Answer from the drawing. Dimensions are ordinates in mm from the lowest x, y and z of the part. A direction names the side the tool comes from. Coordinates: 2 decimals unless noted, no trailing zeros. Write each loop counter-clockwise with the first axis right and the second up, starting at its lowest first coordinate (ties: lowest second). Pieces come first, ordered by that corner, then holes. Notation, with made-up numbers: (10.5, 13) -> (56.5, 13) arc R13 cw to (56.5, 27) -> close; hole circle Ø11 at (16.5, 62.25). An arc over 180 degrees is marked (long way). Return JSON: item names as keys, results as strings.
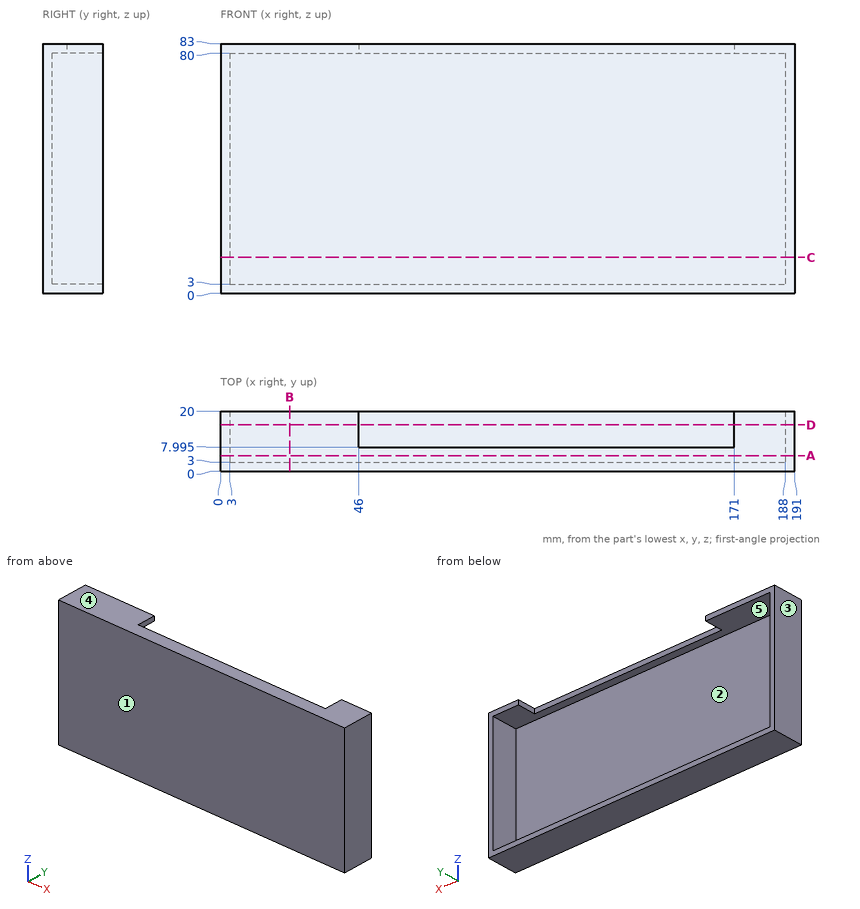
1. The part is cut by section D-D (y = 15.5). Determine the outline of the cut face in (x, z), then the cut area to 3 significant figures.
Taken from the geometry:
{"outline": "(0, 0) -> (191, 0) -> (191, 83) -> (171, 83) -> (171, 80) -> (188, 80) -> (188, 3) -> (3, 3) -> (3, 80) -> (46, 80) -> (46, 83) -> (0, 83) -> close", "area": "1,230 mm2"}
2. The part is cut by section C-C (z = 12). Determine the outline of the cut face in (x, y), then the cut area to 3 significant figures.
Taken from the geometry:
{"outline": "(0, 0) -> (191, 0) -> (191, 20) -> (188, 20) -> (188, 3) -> (3, 3) -> (3, 20) -> (0, 20) -> close", "area": "675 mm2"}
3. The part is cut by section B-B (x = 23). Determine the outline of the cut face in (y, z).
Taken from the geometry:
{"outline": "(0, 0) -> (20, 0) -> (20, 3) -> (3, 3) -> (3, 80) -> (20, 80) -> (20, 83) -> (0, 83) -> close"}
4. For a pull along X with two mould halves and no side action, classify the marked faces 1, 2 and 3 as +X half, -X half, draft (parallel to the pull), parting line (faces both ways), or undercut.
Taken from the geometry:
{"face 1": "draft", "face 2": "undercut", "face 3": "-X half"}
5. A tool of negligible diameter and unlimited length cuts with its end or side. For the marked faces 4 and 5, from which of +Z, -Z, +X, -X, +Y, -Y can it reach the whole face along a straight path? Write none if from no direction.
Taken from the geometry:
{"face 4": "+Z, +X, -X, +Y, -Y", "face 5": "+Y"}
6. Flat-ended cylindrical pins translate along their axes: pin 1 Ø1.5 at (x, z) = (120, 82) entering from +Y (3 decimals); pin 2 Ø12 at (y, z) = (4.5, 27.5) entering from -X; pin 3 Ø1.5 at (x, z) = (143, 65.5) entering from +Y; pin 4 Ø1 at (x, y) = (165.5, 14) entering from +Z. Find the tip coordinate at first contact, or state that the pin passes through.
Taken from the geometry:
{"pin 1": "stops at y = 7.995", "pin 2": "stops at x = 0", "pin 3": "stops at y = 3", "pin 4": "stops at z = 3"}
7. The part is cut by section A-A (y = 5.25). Determine the outline of the cut face in (x, z), then the cut area to 3 significant figures.
Taken from the geometry:
{"outline": "(0, 0) -> (191, 0) -> (191, 83) -> (0, 83) -> close; hole (3, 3) -> (188, 3) -> (188, 80) -> (3, 80) -> close", "area": "1,610 mm2"}
8. Consider L1, parallel to X at y = 10.75, z = 43.5; L2, parallel to Z at x = 43, y = 5.75; L3, parallel to Y at x = 79, z = 15.5. Determine where each line is inside the solid, lowest interval first.
Taken from the geometry:
{"L1": "x = 0 to 3, 188 to 191", "L2": "z = 0 to 3, 80 to 83", "L3": "y = 0 to 3"}
